Verification items for the finished model (mm, model axes). Face numbers are marked on the shaded views. A direction names the side the tool comes from. Give positions to 0.01 mm unless a question says otherwise; leave off trailing zeros. Write each loop counter-clockwise with the first axis right and the second up, starting at its lowest first coordinate (ties: lowest second). Pieces come first, ordered by that corner, then holes. Notation, with made-up numbers: (27, -14) -> (70, -14) arc R22 ccw to (70, 13) -> close; hole circle Ø2 at (76.5, 9.25). An arc over 180 degrees is marked (long way). Use CSV: the item, a comma, the result in double quotes. Start each with the question number.
```python
from build123d import *

# Parameters (mm, degrees)
SKETCH_1_W               = 100.6
SKETCH_1_H               = 25
EXTRUDE_1_DEPTH          = 1
SM_START                 = -12.5
SM_EDGE_FLANGE_1_DEPTH   = 25
SM_EDGE_FLANGE_1_2_DEPTH = 25
SM_EDGE_FLANGE_2_DEPTH   = 25
SM_EDGE_FLANGE_2_2_DEPTH = 25
SKETCH_18_R              = 1.5
CUT_EXTRUDE_1_DEPTH      = 1
SKETCH_19_R              = 1.5
CUT_EXTRUDE_2_DEPTH      = 1
FILLET_1_R               = 2
SKETCH_21_R              = 5
CUT_EXTRUDE_3_DEPTH      = 1
SKETCH_22_R              = 1.5
CUT_EXTRUDE_4_DEPTH      = 10


# Read off the part's stored shape, not the designer's step: Ребро-кромка1, Ребро-кромка2
with BuildPart() as part:
    # Sketch 1 → Бобышка-Вытянуть1 (new body)
    with BuildSketch(Plane(origin=(0, 0, 0), x_dir=(1, 0, 0), z_dir=(0, 1, 0))):
        Rectangle(SKETCH_1_W, SKETCH_1_H)
    extrude(amount=EXTRUDE_1_DEPTH)

    # Ребро-кромка1 outline → Ребро-кромка1 (cut)
    with BuildSketch(Plane.XY.offset(SM_START)):
        with BuildLine():
            Line((-50.3, 0), (-50.29525739, 0.013030215))
            ThreePointArc((-50.29525739, 0.013030215), (-49.746083113, 0.728728066), (-48.885718458, 1))
            Line((-48.885718458, 1), (-50.3, 1))
            Line((-50.3, 1), (-50.3, 0))
        make_face()
        with BuildLine():
            Line((50.3, 1), (48.885718458, 1))
            ThreePointArc((48.885718458, 1), (49.746083113, 0.728728066), (50.29525739, 0.013030215))
            Line((50.29525739, 0.013030215), (50.3, 0))
            Line((50.3, 0), (50.3, 1))
        make_face()
    extrude(amount=SM_EDGE_FLANGE_1_DEPTH, mode=Mode.SUBTRACT)

    # Sm Edge Flange 1 2 outline → Sm Edge Flange 1 2 (add)
    with BuildSketch(Plane.XY.offset(SM_START)):
        with BuildLine():
            Line((-48.885718458, 0), (-50.3, 0))
            Line((-50.3, 0), (-55.066331916, -13.095389312))
            Line((-55.066331916, -13.095389312), (-54.126639295, -13.437409455))
            Line((-54.126639295, -13.437409455), (-49.355564769, -0.328989928))
            ThreePointArc((-49.355564769, -0.328989928), (-49.172506676, -0.090423978), (-48.885718458, 0))
        make_face()
        with BuildLine():
            Line((50.3, 0), (48.885718458, 0))
            ThreePointArc((48.885718458, 0), (49.172506676, -0.090423978), (49.355564769, -0.328989928))
            Line((49.355564769, -0.328989928), (54.126639295, -13.437409455))
            Line((54.126639295, -13.437409455), (55.066331916, -13.095389312))
            Line((55.066331916, -13.095389312), (50.3, 0))
        make_face()
    extrude(amount=SM_EDGE_FLANGE_1_2_DEPTH)

    # Ребро-кромка2 outline → Ребро-кромка2 (cut)
    with BuildSketch(Plane.XY.offset(SM_START)):
        with BuildLine():
            Line((55.066331916, -13.095389312), (55.05246545, -13.095389312))
            ThreePointArc((55.05246545, -13.095389312), (54.192100796, -12.824117378), (53.642926519, -12.108419527))
            Line((53.642926519, -12.108419527), (54.126639295, -13.437409455))
            Line((54.126639295, -13.437409455), (55.066331916, -13.095389312))
        make_face()
        with BuildLine():
            Line((-55.05246545, -13.095389312), (-55.066331916, -13.095389312))
            Line((-55.066331916, -13.095389312), (-54.126639295, -13.437409455))
            Line((-54.126639295, -13.437409455), (-53.642926519, -12.108419527))
            ThreePointArc((-53.642926519, -12.108419527), (-54.192100796, -12.824117378), (-55.05246545, -13.095389312))
        make_face()
    extrude(amount=SM_EDGE_FLANGE_2_DEPTH, mode=Mode.SUBTRACT)

    # Sm Edge Flange 2 2 outline → Sm Edge Flange 2 2 (add)
    with BuildSketch(Plane.XY.offset(SM_START)):
        with BuildLine():
            Line((54.58261914, -11.766399383), (55.066331916, -13.095389312))
            Line((55.066331916, -13.095389312), (64.002154143, -13.095389312))
            Line((64.002154143, -13.095389312), (64.002154143, -12.095389312))
            Line((64.002154143, -12.095389312), (55.05246545, -12.095389312))
            ThreePointArc((55.05246545, -12.095389312), (54.765677232, -12.004965334), (54.58261914, -11.766399383))
        make_face()
        with BuildLine():
            Line((-64.002154143, -12.095389312), (-64.002154143, -13.095389312))
            Line((-64.002154143, -13.095389312), (-55.066331916, -13.095389312))
            Line((-55.066331916, -13.095389312), (-54.58261914, -11.766399383))
            ThreePointArc((-54.58261914, -11.766399383), (-54.765677232, -12.004965334), (-55.05246545, -12.095389312))
            Line((-55.05246545, -12.095389312), (-64.002154143, -12.095389312))
        make_face()
    extrude(amount=SM_EDGE_FLANGE_2_2_DEPTH)

    # Эскиз18 → Вырез-Вытянуть1 (cut)
    with BuildSketch(Plane(origin=(0, 1, 0), x_dir=(1, 0, 0), z_dir=(0, 1, 0))):
        with Locations(Location((-7.285718458, 7.5, 0), (0, 0, 270))):
            Circle(SKETCH_18_R)
        with Locations(Location((-7.285718458, -7.5, 0), (0, 0, 90))):
            Circle(SKETCH_18_R)
    extrude(amount=-CUT_EXTRUDE_1_DEPTH, mode=Mode.SUBTRACT)

    # Эскиз19 → Вырез-Вытянуть2 (cut)
    with BuildSketch(Plane(origin=(0, -12.095389312, 0), x_dir=(1, 0, 0), z_dir=(0, 1, 0))):
        with Locations(Location((59.002154143, 7.5, 0), (0, 0, 270))):
            Circle(SKETCH_19_R)
        with Locations(Location((59.002154143, -7.5, 0), (0, 0, 90))):
            Circle(SKETCH_19_R)
        with Locations(Location((-59.002154143, -7.5, 0), (0, 0, 270))):
            Circle(SKETCH_19_R)
        with Locations(Location((-59.002154143, 7.5, 0), (0, 0, 90))):
            Circle(SKETCH_19_R)
    extrude(amount=-CUT_EXTRUDE_2_DEPTH, mode=Mode.SUBTRACT)

    # Скругление1
    fillet_1_edges = [part.edges().sort_by_distance(p)[0] for p in [
        (64.002154143, -12.595389312, 12.5),
        (64.002154143, -12.595389312, -12.5),
        (-64.002154143, -12.595389312, -12.5),
        (-64.002154143, -12.595389312, 12.5),
    ]]
    fillet(fillet_1_edges, radius=FILLET_1_R)

    # Эскиз21 → Вырез-Вытянуть3 (cut)
    with BuildSketch(Plane(origin=(0, 1, 0), x_dir=(1, 0, 0), z_dir=(0, 1, 0))):
        with Locations(Location((-21.885718458, 0, 0), (0, 0, 270))):
            Circle(SKETCH_21_R)
    extrude(amount=-CUT_EXTRUDE_3_DEPTH, mode=Mode.SUBTRACT)

    # Эскиз22 → Вырез-Вытянуть4 (cut)
    with BuildSketch(Plane(origin=(0, 1, 0), x_dir=(1, 0, 0), z_dir=(0, 1, 0))):
        with Locations(Location((-43.835718458, 0, 0), (0, 0, 270))):
            Circle(SKETCH_22_R)
    extrude(amount=-CUT_EXTRUDE_4_DEPTH, mode=Mode.SUBTRACT)


solid = part.part
```
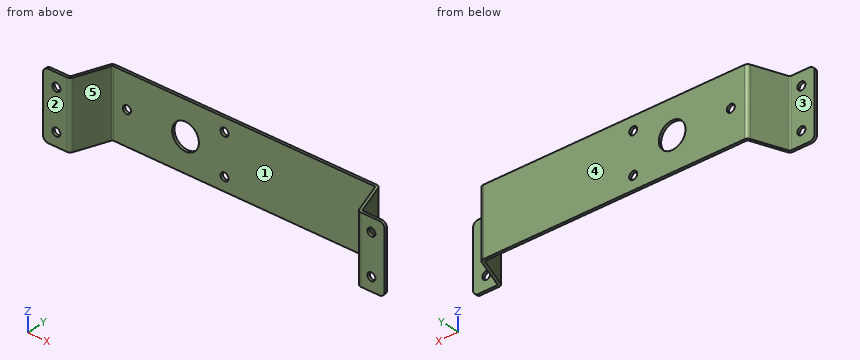
(1) Draft check along X on the marked faces 4 and 5. Enter one of: released by +X, released by -X, zero draft, split by the parting line, or undercut.
(2) Section check C-C on y = -7.5. Record the cut outline in (x, z).
(3) Thickness scan on line 1 (X direction, y = 0.7, z = 0); line 2 (X direction, y = 0.6, z = 0); line 3 (X direction, y = -12.35, z = 7.5). Record the ranges inside material, lowest first. Write a range as from..to.
(4) Go/stop test with flat-tipped pins: pin 1 (7.5 mm diameter, centred on x = -18.5, z = 2.5, fed in from -Y); pin 2 (2.5 mm diameter, centred on x = -59, z = -7.5, fed in from -Y); pin 3 (5 mm diameter, centred on x = -7.29, z = -7.5, fed in from +Y); pin 4 (8 mm diameter, centred on y = -7.5, z = -2.5, fed in from -X). Record where each tip stops, or that it passes through.
(5) Section check A-A on z = -7.5. Give the number of separate pieces and of enclosed holes in the cut face, then the cut area to 3 significant figures.
(6) Section check B-B on z = 0. Record the cut outline in (x, y), then the cut area to 3 significant figures.
(7) Section check D-D on x = 19.5. Record the cut outline in (y, z).
(8) Set-up check for the marked faces 1, 2 and 3: record each of +Z, -Z, +X, -X, +Y, -Y from which the full face is reachable in a straight line by a thin tool's end or side.
Data:
1,face 4,"zero draft"
1,face 5,"undercut"
2,outline,"(-53.03, -12.5) -> (-51.97, -12.5) -> (-51.97, 12.5) -> (-53.03, 12.5) -> close; (51.97, -12.5) -> (53.03, -12.5) -> (53.03, 12.5) -> (51.97, 12.5) -> close"
3,line 1,"x = -49.79..-45.34, -42.34..-26.89, -16.89..49.79"
3,line 2,"x = -49.91..-45.34, -42.34..-26.89, -16.89..49.91"
3,line 3,"x = -64..-60.5, -57.5..-53.76, 53.76..57.5, 60.5..64"
4,pin 1,"stops at y = 0"
4,pin 2,"passes through"
4,pin 3,"stops at y = 1"
4,pin 4,"stops at x = -54.49"
5,separate pieces,"4"
5,enclosed holes,"0"
5,area,"137 mm2"
6,outline,"(-64, -13.1) -> (-55.05, -13.1) arc R1.5 ccw to (-53.64, -12.11) -> (-49.36, -0.33) arc R0.5 cw to (-48.89, 0) -> (-45.34, 0) -> (-45.34, 1) -> (-48.89, 1) arc R1.5 ccw to (-50.3, 0.01) -> (-54.58, -11.77) arc R0.5 cw to (-55.05, -12.1) -> (-64, -12.1) -> close; (-42.34, 0) -> (-26.89, 0) -> (-26.89, 1) -> (-42.34, 1) -> close; (-16.89, 0) -> (48.89, 0) arc R0.5 cw to (49.36, -0.33) -> (53.64, -12.11) arc R1.5 ccw to (55.05, -13.1) -> (64, -13.1) -> (64, -12.1) -> (55.05, -12.1) arc R0.5 cw to (54.58, -11.77) -> (50.3, 0.01) arc R1.5 ccw to (48.89, 1) -> (-16.89, 1) -> close"
6,area,"133 mm2"
7,outline,"(0, -12.5) -> (1, -12.5) -> (1, 12.5) -> (0, 12.5) -> close"
8,face 1,"+Z, -Z, -Y"
8,face 2,"+Z, -Z, +X, -X, -Y"
8,face 3,"+Z, -Z, -X, +Y"
